The model under review builds one solid part; all positions refer to its coordinate system, in mm. Face numbers are marked on the shaded views. A direction names the side the tool comes from. Give positions to 0.01 mm unless a question says otherwise; leave off trailing zeros. Loops run counter-clockwise (first coordinate to the right, second up) from the corner with the lowest first, then second, coordinate; pieces in that order, holes last. Notation, with made-up numbers: M -36,75 L 17,75 A12 ccw 17,98 Z; hole C 27.25,14.5 d1. An arc over 180 degrees is marked long. Write item = value, one per line. Start each with the question number.
1. For pin 1 (4 mm diameter, centred on x = 3, z = -5.5, fed in from +Y); pin 2 (5 mm diameter, centred on y = 7, z = -7, fed in from -X); pin 3 (0.8 mm diameter, centred on y = 8, z = -4, fed in from +X); pin 4 (1.2 mm diameter, centred on x = 0, z = 0, fed in from -Y), all flat-tipped, find the tip position at first contact; note any pin that passes through.
2. We need section D-D on z = 6. Give the boundary of the cut face in (x, y), then the cut area to 3 significant figures.
3. We need section A-A on x = 0. Give the boundary of the cut face in (y, z), then the cut area to 3 significant figures.
4. We need section C-C on x = -6.25. Give the boundary of the cut face in (y, z).
5. Draft analysis for pull direction Z (two halves, no side actions). For the marked faces 6, 7, 8 and 9, state which applies: pulls with the +Z half, pulls with the -Z half, needs draft (parallel to the pull), parting line crosses it, or undercut.
6. Wall thickness on line 1 along X through (y, z) = (5.15, 0); line 2 along Z through (x, y) = (0, 2.85): over which ranges is each line inside the solid? List them lowest first. Write a range as from..to.
7. We need section B-B on z = 0. Give the boundary of the cut face in (x, y).
8. For the marked faces 1, 2, 3, 4 and 5, list the 3-axis set-ups (+Z, -Z, +X, -X, +Y, -Y) from which the entire face can be reached by the end or side of a thin tool; tool diameter is ignored.
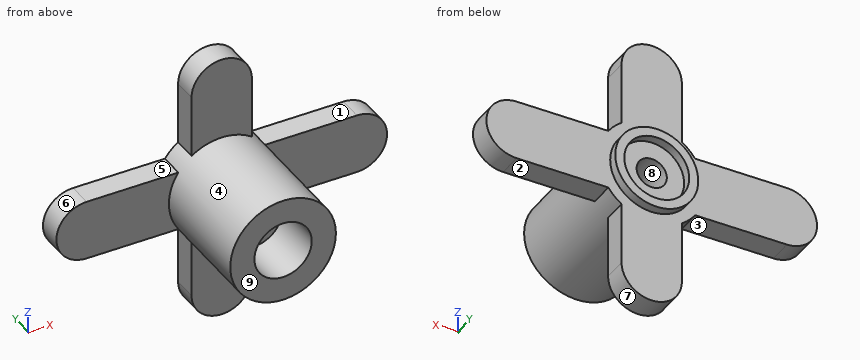
from build123d import *

# Parameters (mm, degrees)
SZKIC1_R                    = 3.5
DODANIE_WYCI_GNI_CIE1_DEPTH = 9.5
SZKIC2_R                    = 1.9
WYTNIJ_WYCI_GNI_CIE1_DEPTH  = 3.5
SZKIC3_R                    = 2
DODANIE_WYCI_GNI_CIE2_DEPTH = 1.6
WYTNIJ_WYCI_GNI_CIE2_START  = -0.6
SZKIC4_R                    = 2.15
WYTNIJ_WYCI_GNI_CIE2_DEPTH  = 0.6
SZKIC5_R                    = 1
WYTNIJ_WYCI_GNI_CIE3_DEPTH  = 31.6
SZKIC6_R                    = 3.5
SZKIC6_R_2                  = 2.75
WYTNIJ_WYCI_GNI_CIE4_DEPTH  = 0.6


with BuildPart() as part:
    # Szkic1 → Dodanie-wyciągnięcie1 (new body)
    with BuildSketch(Plane(origin=(0, 0, 0), x_dir=(1, 0, 0), z_dir=(0, 1, 0))):
        Circle(SZKIC1_R)
    extrude(amount=DODANIE_WYCI_GNI_CIE1_DEPTH)

    # Szkic2 → Wytnij-wyciągnięcie1 (cut)
    with BuildSketch(Plane.XZ):
        Circle(SZKIC2_R)
    extrude(amount=-WYTNIJ_WYCI_GNI_CIE1_DEPTH, mode=Mode.SUBTRACT)

    # Szkic3 → Dodanie-wyciągnięcie2 (add)
    with BuildSketch(Plane(origin=(0, 8.9, 0), x_dir=(1, 0, 0), z_dir=(0, 1, 0))):
        with Locations((-8.95, 0)):
            Circle(SZKIC3_R)
        with BuildLine():
            Line((-2, 2), (-8.95, 2))
            ThreePointArc((-8.95, 2), (-7.535786438, 1.414213562), (-6.95, 0))
            ThreePointArc((-6.95, 0), (-7.535786438, -1.414213562), (-8.95, -2))
            Line((-8.95, -2), (-2, -2))
            Line((-2, -2), (-2, 2))
        make_face()
        with Locations((0, 7)):
            Circle(SZKIC3_R)
        with BuildLine():
            Line((-2, 7), (-2, 2))
            Line((-2, 2), (0, 2))
            Line((0, 2), (2, 2))
            Line((2, 2), (2, 7))
            ThreePointArc((2, 7), (0, 5), (-2, 7))
        make_face()
        with BuildLine():
            Line((8.95, 2), (2, 2))
            Line((2, 2), (2, 0))
            Line((2, 0), (2, -2))
            Line((2, -2), (8.95, -2))
            ThreePointArc((8.95, -2), (6.95, 0), (8.95, 2))
        make_face()
        with Locations((8.95, 0)):
            Circle(SZKIC3_R)
        with Locations((0, -7)):
            Circle(SZKIC3_R)
        with BuildLine():
            Line((2, -2), (-2, -2))
            Line((-2, -2), (-2, -7))
            ThreePointArc((-2, -7), (0, -5), (2, -7))
            Line((2, -7), (2, -2))
        make_face()
    extrude(amount=-DODANIE_WYCI_GNI_CIE2_DEPTH)

    # Szkic4 → Wytnij-wyciągnięcie2 (cut)
    with BuildSketch(Plane(origin=(0, 9.5, 0), x_dir=(1, 0, 0), z_dir=(0, 1, 0)).offset(WYTNIJ_WYCI_GNI_CIE2_START)):
        Circle(SZKIC4_R)
    extrude(amount=WYTNIJ_WYCI_GNI_CIE2_DEPTH, mode=Mode.SUBTRACT)

    # Szkic5 → Wytnij-wyciągnięcie3 (cut)
    with BuildSketch(Plane(origin=(0, 8.9, 0), x_dir=(1, 0, 0), z_dir=(0, 1, 0))):
        Circle(SZKIC5_R)
    extrude(amount=-WYTNIJ_WYCI_GNI_CIE3_DEPTH, mode=Mode.SUBTRACT)

    # Szkic6 → Wytnij-wyciągnięcie4 (cut)
    with BuildSketch(Plane(origin=(0, 9.5, 0), x_dir=(1, 0, 0), z_dir=(0, 1, 0))):
        Circle(SZKIC6_R)
        Circle(SZKIC6_R_2, mode=Mode.SUBTRACT)
    extrude(amount=-WYTNIJ_WYCI_GNI_CIE4_DEPTH, mode=Mode.SUBTRACT)


solid = part.part
Final values:
q1.pin_1 = 8.9
q1.pin_2 = -2
q1.pin_3 = 2
q1.pin_4 = through
q2.outline = M -2,7.3 L 2,7.3 L 2,8.9 L -2,8.9 Z
q2.area = 6.40 mm²
q3.outline = M 0,-3.5 L 7.3,-3.5 L 7.3,-9 L 8.9,-9 L 8.9,-2.75 L 9.5,-2.75 L 9.5,-2.15 L 8.9,-2.15 L 8.9,-1 L 3.5,-1 L 3.5,-1.9 L 0,-1.9 Z; M 0,1.9 L 3.5,1.9 L 3.5,1 L 8.9,1 L 8.9,2.15 L 9.5,2.15 L 9.5,2.75 L 8.9,2.75 L 8.9,9 L 7.3,9 L 7.3,3.5 L 0,3.5 Z
q3.area = 56.5 mm²
q4.outline = M 7.3,-2 L 8.9,-2 L 8.9,2 L 7.3,2 Z
q5.face_6 = parting line crosses it
q5.face_7 = pulls with the -Z half
q5.face_8 = undercut
q5.face_9 = needs draft
q6.line_1 = -3.5..-1, 1..3.5
q6.line_2 = -3.5..-1.9, 1.9..3.5
q7.outline = M -10.95,7.3 L -3.5,7.3 L -3.5,0 L -1.9,0 L -1.9,3.5 L -1,3.5 L -1,8.9 L -2.15,8.9 L -2.15,9.5 L -2.75,9.5 L -2.75,8.9 L -10.95,8.9 Z; M 1,3.5 L 1.9,3.5 L 1.9,0 L 3.5,0 L 3.5,7.3 L 10.95,7.3 L 10.95,8.9 L 2.75,8.9 L 2.75,9.5 L 2.15,9.5 L 2.15,8.9 L 1,8.9 Z
q8.face_1 = +Z, +X, +Y, -Y
q8.face_2 = -Z, +X, +Y, -Y
q8.face_3 = -Z, -X, +Y, -Y
q8.face_4 = -Y
q8.face_5 = +Z, -X, +Y, -Y
